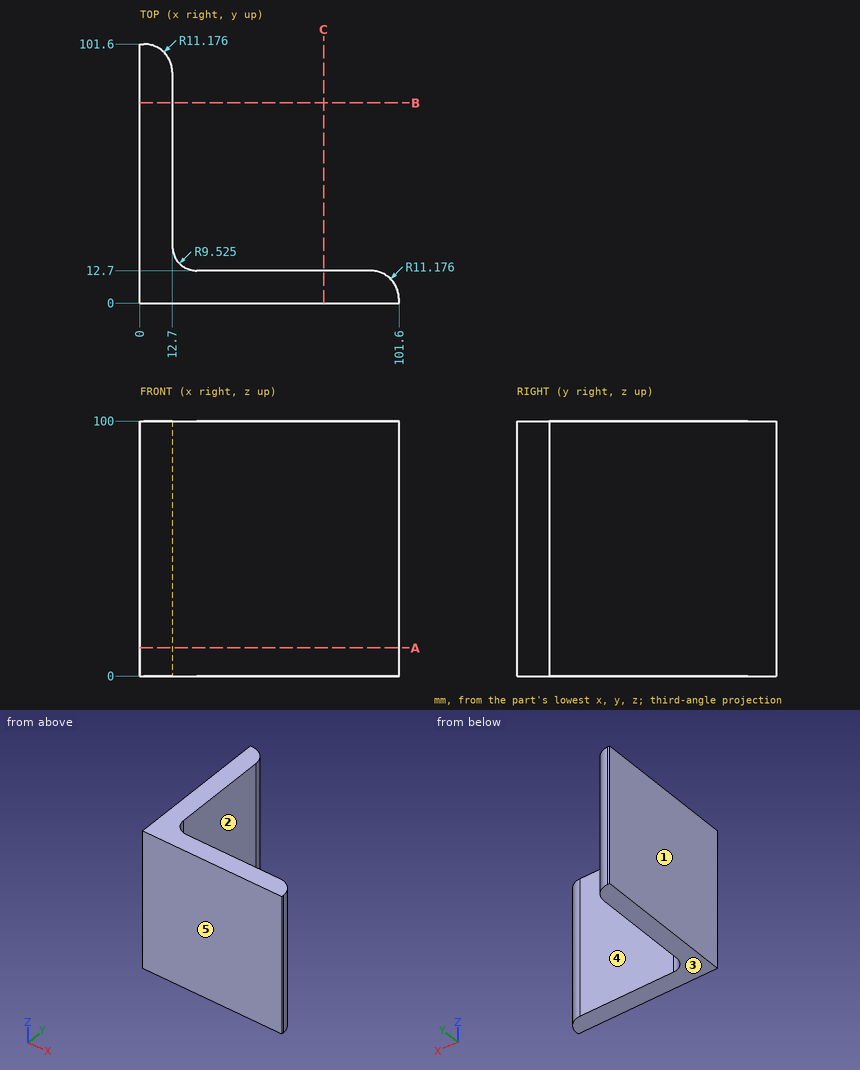
Part print with two shaded views. Sizes in mm from the minimum x, y, z corner. A direction names the side the tool comes from. Give positions to 0.01 mm unless a question says otherwise; leave off trailing zeros. Write each loop counter-clockwise with the first axis right and the second up, starting at its lowest first coordinate (ties: lowest second). Pieces come first, ordered by that corner, then holes.
1) Pin check, flat tips, straight feed: pin 1 (20.5 mm diameter, centred on y = 53, z = 74.5, fed in from +X); pin 2 (1.5 mm diameter, centred on x = 37, z = 54, fed in from +Y). Stop position of each tip, or through.
Resolved:
pin 1: stops at x = 12.7
pin 2: stops at y = 12.7
2) Cut at B-B on y = 78.5. Write the cut outline in (x, z), then the cut area to 3 significant figures.
Resolved:
outline: (0, 0) - (12.7, 0) - (12.7, 100) - (0, 100) - close
area: 1,270 mm2
3) Cut at A-A on z = 11. Write the cut outline in (x, y) (3 decimals), then the cut area to 3 significant figures.
Resolved:
outline: (0, 0) - (101.6, 0) - (101.6, 1.524) arc R11.176 ccw to (90.424, 12.7) - (22.225, 12.7) arc R9.525 cw to (12.7, 22.225) - (12.7, 90.424) arc R11.176 ccw to (1.524, 101.6) - (0, 101.6) - close
area: 2,390 mm2
4) Two-plate mould, pull along X, no slides. Class the marked faces 1, 2 and 3: released by +X, released by -X, zero draft, split by the parting line, or undercut.
Resolved:
face 1: released by -X
face 2: released by +X
face 3: zero draft
5) Probe L1, parallel to X at y = 78, z = 83; L2, parallel to Y at x = 97, z = 85. List the from-to ranges inside material, lowest first.
Resolved:
L1: x = 0 to 12.7
L2: y = 0 to 10.56
6) Which spindle directions (+Z, -Z, +X, -X, +Y, -Y) get a long thin tool onto all of the face, cutting with end or side? Do the marked faces 4 and 5. Say none if no direction does.
Resolved:
face 4: +Z, -Z, +X, +Y
face 5: +Z, -Z, +X, -X, -Y
